The drawing under review shows one solid part. Ordinate dimensions are in mm from its lowest x, y, z. A direction names the side the tool comes from. Coordinates: 2 decimals unless noted, no trailing zeros. Write each loop counter-clockwise with the first axis right and the second up, starting at its lowest first coordinate (ties: lowest second). Pieces come first, ordered by that corner, then holes.
1) We need section B-B on y = 127. Write out the cut boundary in (x, z) (1 decimal), then the cut area to 3 significant figures.
2) For the marked faces 1 and 2, list the 3-axis set-ups (+Z, -Z, +X, -X, +Y, -Y) from which the entire face can be reached by the end or side of a thin tool; tool diameter is ignored.
3) We need section C-C on z = 7. Write out the cut boundary in (x, y) (1 decimal).
4) We need section D-D on z = 38.1. Give the number of separate pieces and of enclosed holes in the cut face, then the cut area to 3 significant figures.
5) We need section A-A on x = 15. Write out the cut boundary in (y, z) (1 decimal).
6) To check wall thickness, follow line 1 along Y through (x, z) = (49, 38); line 2 along Y through (x, z) = (25.4, 48.55) (1 decimal); line 3 along Z through (x, y) = (0.95, 152.4). State the ranges of each line that lie inside material, in increasing order.
7) Mouldability with a two-part tool opening along X and no side actions: class the marked faces 3, 4 and 5 as pulls with the +X half, pulls with the -X half, needs draft (parallel to the pull), parting line crosses it, or undercut.
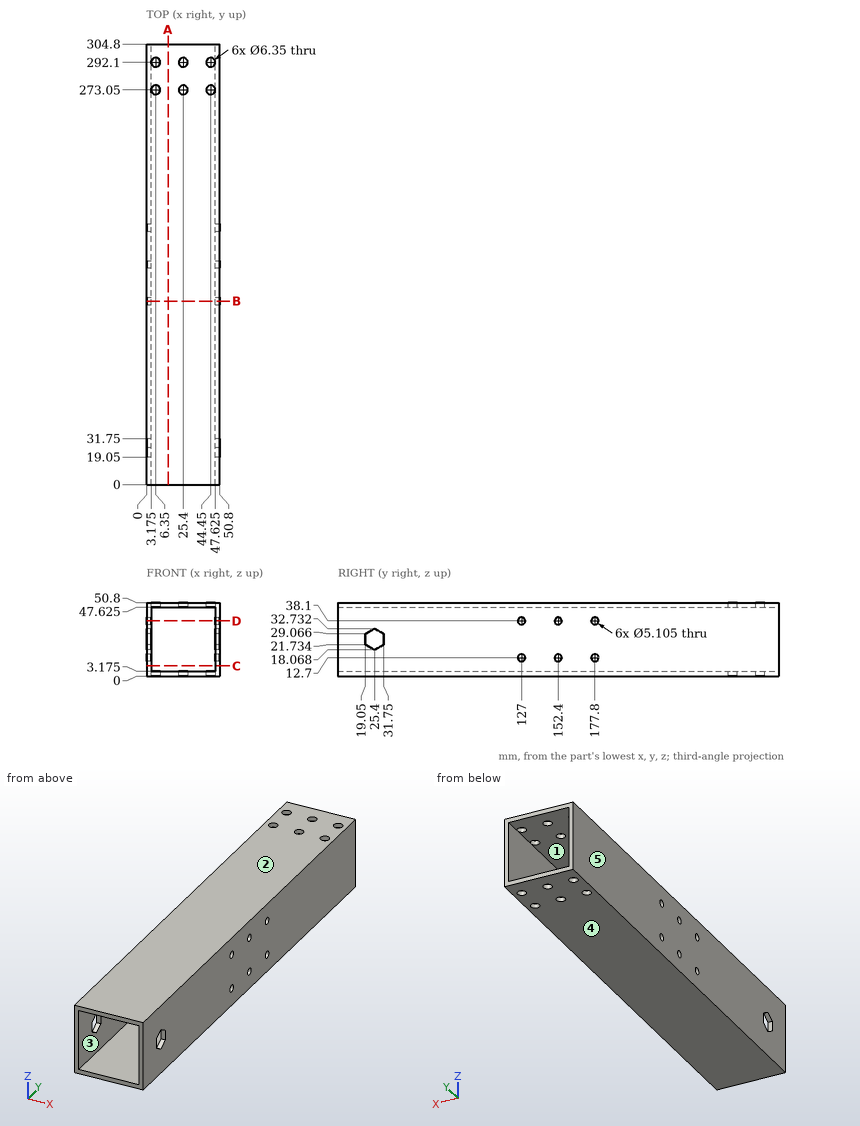
Result:
1. outline: (0, 0) - (50.8, 0) - (50.8, 10.1) - (47.6, 10.1) - (47.6, 3.2) - (3.2, 3.2) - (3.2, 10.1) - (0, 10.1) - close; (0, 15.3) - (3.2, 15.3) - (3.2, 35.5) - (0, 35.5) - close; (0, 40.7) - (3.2, 40.7) - (3.2, 47.6) - (47.6, 47.6) - (47.6, 40.7) - (50.8, 40.7) - (50.8, 50.8) - (0, 50.8) - close; (47.6, 15.3) - (50.8, 15.3) - (50.8, 35.5) - (47.6, 35.5) - close
1. area: 540 mm2
2. face 1: +Y, -Y
2. face 2: +Z, +X, -X, +Y, -Y
3. outline: (0, 0) - (3.2, 0) - (3.2, 304.8) - (0, 304.8) - close; (47.6, 0) - (50.8, 0) - (50.8, 304.8) - (47.6, 304.8) - close
4. separate pieces: 8
4. enclosed holes: 0
4. area: 1,840 mm2
5. outline: (0, 0) - (304.8, 0) - (304.8, 3.2) - (0, 3.2) - close; (0, 47.6) - (304.8, 47.6) - (304.8, 50.8) - (0, 50.8) - close
6. line 1: y = 0 to 124.45, 129.55 to 149.85, 154.95 to 175.25, 180.35 to 304.8
6. line 2: y = 0 to 269.9, 276.2 to 288.9, 295.3 to 304.8
6. line 3: z = 0 to 10.15, 15.25 to 35.55, 40.65 to 50.8
7. face 3: undercut
7. face 4: needs draft
7. face 5: pulls with the -X half
